The listing builds one solid part. Answer for the finished solid, in the listing's coordinates (mm). Give positions to 0.01 mm unless a question says otherwise; leave off trailing zeros. Order: outer loops, then holes, each group sorted by start corner. A loop starts at its lowest first (then second) coordinate and runs counter-clockwise, first axis right, second up.
```python
from build123d import *

# Parameters (mm, degrees)
SKETCH3_W           = 180
SKETCH3_H           = 180
SKETCH3_R           = 50.129190947
SKETCH3_R_2         = 1.47
BOSS_EXTRUDE1_DEPTH = 3.18
CUT_EXTRUDE1_DEPTH  = 128.318939675
SKETCH5_R           = 1.436023081
SKETCH5_W           = 3.18
SKETCH5_H           = 80.125
CUT_EXTRUDE2_DEPTH  = 128.318939675


with BuildPart() as part:
    # Sketch3 → Boss-Extrude1 (new body)
    with BuildSketch(Plane.XY):
        Rectangle(SKETCH3_W, SKETCH3_H)
        with Locations(Location((0, 0, 0), (0, 0, 180))):
            Circle(SKETCH3_R, mode=Mode.SUBTRACT)
        with Locations(Location((-48.029419272, 24.129595611, 0), (0, 0, 180))):
            Circle(SKETCH3_R_2, mode=Mode.SUBTRACT)
        with Locations(Location((-24.129595611, -48.029419272, 0), (0, 0, 180))):
            Circle(SKETCH3_R_2, mode=Mode.SUBTRACT)
        with Locations(Location((48.029419272, -24.129595611, 0), (0, 0, 180))):
            Circle(SKETCH3_R_2, mode=Mode.SUBTRACT)
        with Locations(Location((24.129595611, 48.029419272, 0), (0, 0, 180))):
            Circle(SKETCH3_R_2, mode=Mode.SUBTRACT)
    extrude(amount=BOSS_EXTRUDE1_DEPTH)

    # Sketch4 → Cut-Extrude1 (cut, through all)
    with BuildSketch(Plane.XY.offset(3.18)):
        Polygon((1.5, 86.82), (10, 86.82), (10, 90), (-10, 90), (-10, 86.82), (-1.5, 86.82), (-1.5, 82.82), (-3.5, 82.82), (-3.5, 79.82), (-1.5, 79.82), (-1.5, 77), (1.5, 77), (1.5, 79.82), (3.5, 79.82), (3.5, 82.82), (1.5, 82.82), align=None)
        Polygon((1.5, -79.82), (1.5, -77), (-1.5, -77), (-1.5, -79.82), (-3.5, -79.82), (-3.5, -82.82), (-1.5, -82.82), (-1.5, -86.82), (-10, -86.82), (-10, -90), (10, -90), (10, -86.82), (1.5, -86.82), (1.5, -82.82), (3.5, -82.82), (3.5, -79.82), align=None)
    extrude(amount=-CUT_EXTRUDE1_DEPTH, mode=Mode.SUBTRACT)

    # Sketch5 → Cut-Extrude2 (cut, through all)
    with BuildSketch(Plane.XY.offset(3.18)):
        with Locations((-88, 0)):
            Circle(SKETCH5_R)
        with Locations((88, 0)):
            Circle(SKETCH5_R)
        with Locations((-88.41, 49.9375)):
            Rectangle(SKETCH5_W, SKETCH5_H)
        with Locations((-88.41, -49.9375)):
            Rectangle(SKETCH5_W, SKETCH5_H)
        with Locations((88.41, -49.9375)):
            Rectangle(SKETCH5_W, SKETCH5_H)
        with Locations((88.41, 49.9375)):
            Rectangle(SKETCH5_W, SKETCH5_H)
    extrude(amount=-CUT_EXTRUDE2_DEPTH, mode=Mode.SUBTRACT)


solid = part.part
```
1) Find section C-C (y = 67). Write down the section's boundary in (x, z), then the cut area to 3 significant figures.
Geometry says:
outline: (-86.82, 0) - (86.82, 0) - (86.82, 3.18) - (-86.82, 3.18) - close
area: 552 mm2
2) Find section B-B (y = -38). Write down the section's boundary in (x, z).
Geometry says:
outline: (-86.82, 0) - (-32.69, 0) - (-32.69, 3.18) - (-86.82, 3.18) - close; (32.69, 0) - (86.82, 0) - (86.82, 3.18) - (32.69, 3.18) - close
3) Find section D-D (z = 1.15). Count the separate pieces of the cut face and the enclosed holes in it, then the cut area to 3 significant figures.
Geometry says:
separate pieces: 1
enclosed holes: 7
area: 23,200 mm2
4) Find section A-A (x = -19.5). Write down the section's boundary in (y, z).
Geometry says:
outline: (-90, 0) - (-46.18, 0) - (-46.18, 3.18) - (-90, 3.18) - close; (46.18, 0) - (90, 0) - (90, 3.18) - (46.18, 3.18) - close
5) For a pull along Y with two mould halves and no side action, classify faces 1 (the cylindrical face through (-47.8, -15.1, 1.6)), 2 (the flat face through (-41, 41, 3.18)) as +Y half, -Y half, draft (parallel to the pull), parting line (faces both ways), or undercut.
Geometry says:
face 1: undercut
face 2: draft
6) Given P1, Ø2.5, axis at x = 88, y = 0, coming from the +Z side (1 decimal); P2, Ø1.6, axis at y = -84.5, z = 2, coming from the -X side; P3, Ø1, axis at x = 88, z = 1, coming from the -Y side (3 decimals); P4, Ø1.5, axis at y = 81.5, z = 1.5, coming from the +X side, each flat-ended and moving along its own axis, determine where each tip first touches the part or whether it passes through.
Geometry says:
P1: passes through
P2: stops at x = -86.82
P3: stops at y = -9.875
P4: stops at x = 86.82
7) Straight lines are drawn through the part: probe 1 along Y at (x, z) = (-1, 0.55); probe 2 along X at (y, z) = (-81.5, 0.45); probe 3 along Y at (x, z) = (43.5, 0.55). For each, find the intervals that lie inside material, in ascending order.
Geometry says:
probe 1: y = -77 to -50.12, 50.12 to 77
probe 2: x = -86.82 to -3.5, 3.5 to 86.82
probe 3: y = -90 to -24.91, 24.91 to 90
